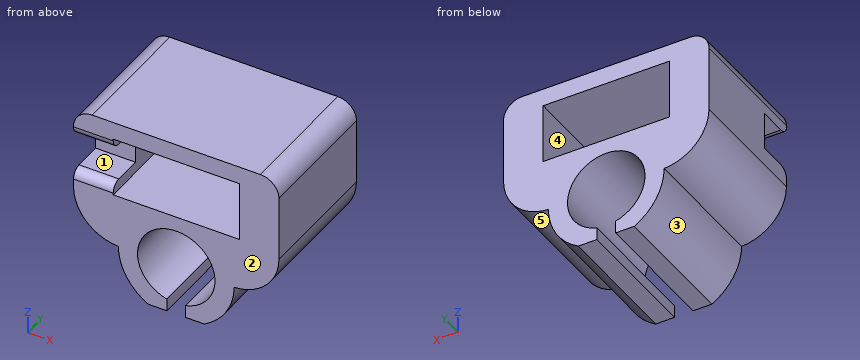
Solid Edge part; units mm, degrees
sketch "Sketch1" plane through (0, 0, 0) normal (0, -1, 0) x (1, 0, 0)
  line L0 (-6.75, -4.3) -> (6.75, -4.3)
  line L1 (6.75, -4.3) -> (6.75, 2.1)
  line L2 (6.75, 2.1) -> (-6.75, 2.1)
  line L3 (-6.75, 2.1) -> (-6.75, -4.3)
  line L4 (11, -5) -> (11, 4)
  line L5 (11, 4) -> (-11, 4)
  line L6 (-11, 4) -> (-11, -5)
  arc A0 (-11, -5) -> (-6.2, -10) centre (-5.9958, -5) ccw
  line L7 (-3, -15.4259) -> (-1, -15.4259)
  line L8 (-1, -14.0792) -> (-1, -15.4259)
  line L9 (1, -15.4259) -> (1, -14.0792)
  line L10 (3, -15.4259) -> (1, -15.4259)
  arc A1 (6.2, -10) -> (3, -15.4259) centre (0, -10) cw
  arc A2 (11, -5) -> (6.2, -10) centre (5.9958, -5) cw
  arc A3 (-6.2, -10) -> (-3, -15.4259) centre (0, -10) ccw
  arc A4 (-1, -14.0792) -> (1, -14.0792) centre (0, -10.0515) cw
extrude "Protrusion1" add sketch "Sketch1" against normal blind 14
sketch "Sketch2" plane through (0, 0, -5.7129) normal (0, -1, 0) x (1, 0, 0)
  line L0 (-11.9165, 2.6129) -> (-5.9165, 2.6129)
  line L1 (-5.9165, 2.6129) -> (-5.9165, 6.6129)
  line L2 (-5.9165, 6.6129) -> (-11.9165, 6.6129)
  line L3 (-11.9165, 6.6129) -> (-11.9165, 2.6129)
extrude "ExtrudedCutout_2" cut sketch "Sketch2" against normal blind 4
fillet "Round_2" radius 1 2 edges at (-8.875, 0, 0.9) (-8.875, 0, -3.1)
fillet "Round_3" radius 2 2 edges at (-11, 7, 4) (11, 7, 4)
The listing builds one solid part. Answer for the finished solid, in the listing's coordinates (mm). Face numbers are marked on the shaded views. A direction names the side the tool comes from. Give positions to 0.01 mm unless a question says otherwise; leave off trailing zeros. Order: outer loops, then holes, each group sorted by start corner. A loop starts at its lowest first (then second) coordinate and runs counter-clockwise, first axis right, second up. Notation, with made-up numbers: (4.5, 17.25) - (33.5, 17.25) arc R22 cw to (33.5, 42.25) - close; hole circle Ø2 at (65.5, 30.5). An arc over 180 degrees is marked (long way). Answer as CSV lines item,"result".
Q1. Determine the mould class of the marked faces 1, 2 and 3 for opening direction Z: pulls with the +Z half, pulls with the -Z half, needs draft (parallel to the pull), parting line crosses it, or undercut.
Answer key:
face 1,"undercut"
face 2,"needs draft"
face 3,"pulls with the -Z half"
Q2. A cutting plane is placed at A-A, the plane x = 0. Determine the outline of the cut face in (y, z).
Answer key:
outline,"(0, -5.9) - (14, -5.9) - (14, -4.3) - (0, -4.3) - close; (0, 2.1) - (14, 2.1) - (14, 4) - (0, 4) - close"
Q3. A cutting plane is placed at D-D, the plane x = 9.5. Determine the outline of the cut face in (y, z), and give its area (3 significant figures).
Answer key:
outline,"(0, -8.57) - (14, -8.57) - (14, 3.94) - (0, 3.94) - close"
area,"175 mm^2"
Q4. A cutting plane is placed at C-C, the plane z = -7. Determine the outline of the cut face in (x, y), and give its area (3 significant figures).
Answer key:
outline,"(-10.58, 0) - (-2.81, 0) - (-2.81, 14) - (-10.58, 14) - close; (2.81, 0) - (10.58, 0) - (10.58, 14) - (2.81, 14) - close"
area,"218 mm^2"
Q5. Straight lines are drawn through the part: L1, parallel to X at y = 5.5, z = -0.25; L2, parallel to X at y = 2, z = -10.25; L3, parallel to Z at x = -3.25, y = 8.5. For each, find the intervals that lie inside material, in ascending order.
Answer key:
L1,"x = -11 to -6.75, 6.75 to 11"
L2,"x = -6.19 to -4.15, 4.15 to 6.19"
L3,"z = -15.28 to -12.63, -7.47 to -4.3, 2.1 to 4"
Q6. A cutting plane is placed at B-B, the plane y = 4.75. Determine the outline of the cut face in (x, z).
Answer key:
outline,"(-11, -5) arc R5 ccw to (-6.2, -10) arc R6.2 ccw to (-3, -15.43) - (-1, -15.43) - (-1, -14.08) arc R4.15 cw (long way) to (1, -14.08) - (1, -15.43) - (3, -15.43) arc R6.2 ccw to (6.2, -10) arc R5 ccw to (11, -5) - (11, 2) arc R2 ccw to (9, 4) - (-9, 4) arc R2 ccw to (-11, 2) - close; hole (-6.75, -4.3) - (6.75, -4.3) - (6.75, 2.1) - (-6.75, 2.1) - close"
Q7. Which of the six approach directions +Z, -Z, +X, -X, +Y, -Y give full straight-line access (tool end or side, diameter ignored) to the marked faces 4 and 5?
Answer key:
face 4,"+Y, -Y"
face 5,"-Z, +X, +Y, -Y"
Q8. Each of these flat-tipped pins is pushed along its axis until it touches: pin 1 Ø3 at (y, z) = (6.5, -13) entering from +X; pin 2 Ø5 at (y, z) = (10.5, -8) entering from +X; pin 3 Ø1.1 at (y, z) = (10.5, -15) entering from +X. Where does it stop, or does it pass through?
Answer key:
pin 1,"stops at x = 6.02"
pin 2,"stops at x = 10.97"
pin 3,"stops at x = 4.32"
